from build123d import *

# Parameters (mm, degrees)
SKETCH_1_W      = 27
SKETCH_1_H      = 34
SKETCH_1_R      = 1.75
EXTRUDE_1_DEPTH = 1
EXTRUDE_2_DEPTH = 10
SKETCH_4_R      = 4
EXTRUDE_3_DEPTH = 6
FILLET_1_R      = 1


with BuildPart() as part:
    # 草图1 → 凸台-拉伸1 (new body)
    with BuildSketch(Plane.XY):
        Rectangle(SKETCH_1_W, SKETCH_1_H)
        with Locations((10, 13)):
            Circle(SKETCH_1_R, mode=Mode.SUBTRACT)
        with Locations(Location((-10, 13, 0), (0, 0, 180))):
            Circle(SKETCH_1_R, mode=Mode.SUBTRACT)
        with Locations(Location((10, -13, 0), (0, 0, 180))):
            Circle(SKETCH_1_R, mode=Mode.SUBTRACT)
        with Locations((-10, -13)):
            Circle(SKETCH_1_R, mode=Mode.SUBTRACT)
    extrude(amount=EXTRUDE_1_DEPTH)

    # 草图2 → 凸台-拉伸2 (add)
    with BuildSketch(Plane(origin=(0, 0, 0), x_dir=(-1, 0, 0), z_dir=(0, 0, -1))):
        Polygon((12, 0), (12, 3.5), (9.5, 3.5), (9.5, 6), (-1.5, 6), (-1.5, 3.5), (-4, 3.5), (-4, -3.5), (-1.5, -3.5), (-1.5, -6), (9.5, -6), (9.5, -3.5), (12, -3.5), align=None)
    extrude(amount=EXTRUDE_2_DEPTH)

    # 草图3 → 旋转1 (revolve)
    with BuildSketch(Plane(origin=(-1, 0, 0), x_dir=(0, 0, -1), z_dir=(1, 0, 0))):
        with BuildLine():
            Line((10, -13), (10, 0))
            Line((10, 0), (18.803847577, 0))
            ThreePointArc((18.803847577, 0), (16.395787318, -7.850282354), (10, -13))
        make_face()
    revolve(axis=Axis((-1, 0, -17.702001311), (0, 0, 1)))

    # 草图4 → 凸台-拉伸3 (add)
    with BuildSketch(Plane.XY.offset(-18)):
        with Locations((-1, 0)):
            Circle(SKETCH_4_R)
    extrude(amount=-EXTRUDE_3_DEPTH)

    # 草图5 → 旋转3 (revolve)
    with BuildSketch(Plane(origin=(-1, 0, 0), x_dir=(0, 0, -1), z_dir=(1, 0, 0)), mode=Mode.PRIVATE) as revolve_3_sk:
        with BuildLine():
            Line((24, 0), (24, -8.8))
            ThreePointArc((24, -8.8), (24.807839272, -8.723517815), (25.5, -8.3))
            ThreePointArc((25.5, -8.3), (26.666937336, -4.225350121), (27, 0))
            Line((27, 0), (24, 0))
        make_face()
    revolve(revolve_3_sk.sketch.rotate(Axis((-1, 0, -28.967381471), (0, 0, 1)), 270), axis=Axis((-1, 0, -28.967381471), (0, 0, 1)))

    # 圆角1
    fillet_1_edges = [part.edges().sort_by_distance(p)[0] for p in [
        (7.3, 0, -25.5),
    ]]
    fillet(fillet_1_edges, radius=FILLET_1_R)


solid = part.part
Here's how the part is built. I have some questions about the finished solid (model axes, mm). A direction names the side the tool comes from. Round coordinates to 2 decimals unless told otherwise and drop trailing zeros. Write each loop counter-clockwise with the first axis right and the second up, starting at its lowest first coordinate (ties: lowest second). Pieces come first, ordered by that corner, then holes.
1. For faces 1 (the flat face through (3, 3.5, -5)), 2 (the cylindrical face through (-1.867, -3.905, -21.07)), 3 (the flat face through (3, -3.5, -5)), 4 (the flat face through (-9.5, -5, -5)), 5 (the flat face through (4, 0, -5)), which set-ups out of +Z, -Z, +X, -X, +Y, -Y let a thin tool reach every point of the face, with its end or its side?
2. Will these pins go through, and if not, where does the flat tip stop? pin 1 Ø5 at (x, z) = (-4.5, -5.5) entering from -Y; pin 2 Ø1.1 at (y, z) = (4.5, 0.5) entering from -X; pin 3 Ø5.5 at (x, y) = (-10, -13) entering from -Z; pin 4 Ø2 at (x, y) = (-10, 13) entering from -Z.
3. I need wall thicknesses on L1, parallel to Y at x = 10, z = 0.3; L2, parallel to Y at x = -7.75, z = -6.75; L3, parallel to Z at x = 0.5, y = -8. Which ranges of each line are inside material? Lowest first, please.
4. Suppose I cut it at A-A (y = -12.5). List the corners of the cut face in (x, z) for me, and give its area (3 significant figures).
5. If we mould it in two halves opening along Z, with no side actions, what happens to faces 6 (the cylindrical face through (-10.9, 11.5, 0.5)), 7 (the flat face through (-12, 0, -5)), 8 (the flat face through (0, 0, 1))? For each: released by +Z, released by -Z, zero draft, split by the parting line, or undercut.
6. Suppose I cut it at B-B (z = -2.25). List the corners of the cut face in (x, y) for me, and give its area (3 significant figures).
7. Suppose I cut it at D-D (x = 10). List the corners of the cut face in (y, z) for me.
8. Suppose I cut it at C-C (x = -11). List the corners of the cut face in (y, z) for me, and give its area (3 significant figures).
Answer sheet:
1. face 1: +X, +Y
1. face 2: none
1. face 3: +X, -Y
1. face 4: -X, -Y
1. face 5: +X, +Y, -Y
2. pin 1: stops at y = -6
2. pin 2: stops at x = -13.5
2. pin 3: stops at z = 0
2. pin 4: passes through
3. L1: y = -17 to -14.75, -11.25 to 11.25, 14.75 to 17
3. L2: y = -6 to 6
3. L3: z = -25.56 to -24, -16.19 to -10, 0 to 1
4. outline: (-13.5, 0) - (-11.68, 0) - (-11.68, 1) - (-13.5, 1) - close; (-8.32, 0) - (8.32, 0) - (8.32, 1) - (-8.32, 1) - close; (-4.57, -10) arc R6.3 ccw to (2.57, -10) - close; (11.68, 0) - (13.5, 0) - (13.5, 1) - (11.68, 1) - close
4. area: 25.7 mm2
5. face 6: zero draft
5. face 7: undercut
5. face 8: released by +Z
6. outline: (-12, -3.5) - (-9.5, -3.5) - (-9.5, -6) - (1.5, -6) - (1.5, -3.5) - (4, -3.5) - (4, 3.5) - (1.5, 3.5) - (1.5, 6) - (-9.5, 6) - (-9.5, 3.5) - (-12, 3.5) - close
6. area: 167 mm2
7. outline: (-17, 0) - (-14.75, 0) - (-14.75, 1) - (-17, 1) - close; (-11.25, 0) - (11.25, 0) - (11.25, 1) - (-11.25, 1) - close; (-6.93, -10) arc R8.66 ccw to (6.93, -10) - close; (14.75, 0) - (17, 0) - (17, 1) - (14.75, 1) - close
8. outline: (-17, 0) - (-14.44, 0) - (-14.44, 1) - (-17, 1) - close; (-11.56, 0) - (-3.5, 0) - (-3.5, -10) - (-8.31, -10) arc R9.8 ccw to (8.31, -10) - (3.5, -10) - (3.5, 0) - (11.56, 0) - (11.56, 1) - (-11.56, 1) - close; (14.44, 0) - (17, 0) - (17, 1) - (14.44, 1) - close
8. area: 152 mm2
